Source: CAD feature listing. Evaluate the final solid. Frame: model axes, mm. Round coordinates to 2 decimals unless told otherwise and drop trailing zeros. Write each loop counter-clockwise with the first axis right and the second up, starting at its lowest first coordinate (ties: lowest second). Pieces come first, ordered by that corner, then holes. Notation, with made-up numbers: M -6.75,71.25 L 32.25,71.25 A8 ccw 32.25,78.25 Z; hole C 55,15.25 d11. An arc over 180 degrees is marked long. Answer in a Markdown table with one row per item.
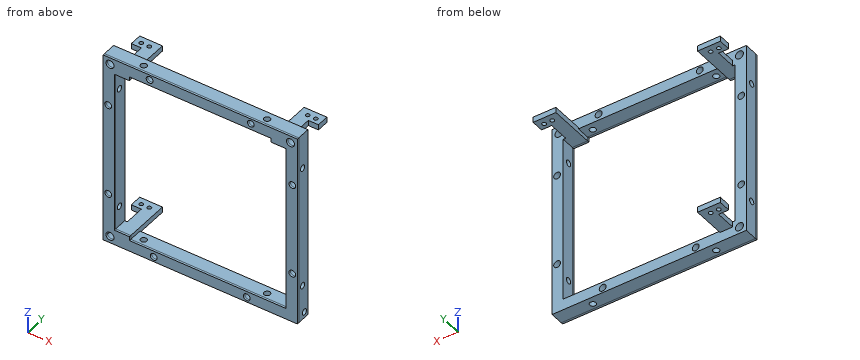
from build123d import *
from build123d.topology import SkipClean

# Parameters (mm, degrees)
SKETCH1_W                       = 96
SKETCH1_H                       = 96
SKETCH1_W_2                     = 80
SKETCH1_H_2                     = 80
BOSS_EXTRUDE1_DEPTH             = 8
SKETCH27_W                      = 82
SKETCH27_H                      = 82
CUT_EXTRUDE2_DEPTH              = 10
F_3_0_3_DIAMETER_HOLE1_D        = 3
F_3_4_3_4_DIAMETER_HOLE1_D      = 3.4
SKETCH38_W                      = 85
SKETCH38_H                      = 85
CUT_EXTRUDE4_DEPTH              = 10
F_3_0_3_DIAMETER_HOLE7_D        = 3
SKETCH44_W                      = 4
SKETCH44_H                      = 4
BOSS_EXTRUDE2_DEPTH             = 8
SKETCH45_W                      = 4
SKETCH45_H                      = 3.5
BOSS_EXTRUDE3_DEPTH             = 8
SKETCH49_W                      = 96
SKETCH49_H                      = 1.5
CUT_EXTRUDE5_DEPTH              = 146
TAP_DRILL_FOR_M4_TAP1_D         = 4
SKETCH53_W                      = 4
SKETCH53_H                      = 6.5
BOSS_EXTRUDE5_DEPTH             = 78
SKETCH57_W                      = 4
SKETCH57_H                      = 6.5
CUT_EXTRUDE6_DEPTH              = 7.5
SKETCH58_W                      = 4
SKETCH58_H                      = 6.5
BOSS_EXTRUDE7_DEPTH             = 81
SKETCH61_W                      = 32
SKETCH61_H                      = 85
CUT_EXTRUDE7_DEPTH              = 81
SKETCH66_W                      = 85
SKETCH66_H                      = 80.198
CUT_EXTRUDE8_DEPTH              = 10
SKETCH67_W                      = 85
SKETCH67_H                      = 85
CUT_EXTRUDE9_DEPTH              = 3.5
SKETCH68_W                      = 52
SKETCH68_H                      = 85
CUT_EXTRUDE10_DEPTH             = 56
SKETCH54_W                      = 6.25
SKETCH54_H                      = 2.7
BOSS_EXTRUDE8_DEPTH             = 16
CUT_EXTRUDE12_START             = -10.22
SKETCH75_W                      = 2.401
SKETCH75_H                      = 3
CUT_EXTRUDE12_DEPTH             = 72.44
SKETCH77_W                      = 2.401
SKETCH77_H                      = 3
CUT_EXTRUDE13_DEPTH             = 6.28
SKETCH78_W                      = 85
SKETCH78_H                      = 85
CUT_EXTRUDE14_DEPTH             = 6.5
SKETCH79_W                      = 85
SKETCH79_H                      = 85
SKETCH79_W_2                    = 81
SKETCH79_H_2                    = 81
BOSS_EXTRUDE12_DEPTH            = 6.5
SKETCH81_W                      = 2.7
SKETCH81_H                      = 6
BOSS_EXTRUDE13_DEPTH            = 5
TAP_DRILL_FOR_M2_TAP1_D         = 2
TAP_DRILL_FOR_M2_TAP1_DEPTH     = 5.5
TAP_DRILL_FOR_M2_TAP2_D         = 2
TAP_DRILL_FOR_M2_TAP2_DEPTH     = 5.5
TAP_DRILL_FOR_M3X0_5_TAP1_D     = 3
TAP_DRILL_FOR_M3X0_5_TAP1_DEPTH = 7.5
SKETCH88_W                      = 2
SKETCH88_H                      = 70
SKETCH88_W_2                    = 70
SKETCH88_H_2                    = 2
CUT_EXTRUDE15_DEPTH             = 10
SKETCH89_W                      = 85
SKETCH89_H                      = 81
CUT_EXTRUDE16_DEPTH             = 10
SKETCH90_W                      = 2
SKETCH90_H                      = 6.5
CUT_EXTRUDE17_DEPTH             = 7.5
SKETCH91_W                      = 96
SKETCH91_H                      = 96
SKETCH91_R                      = 1.7
SKETCH91_R_2                    = 1.64536441
SKETCH91_R_3                    = 2
BOSS_EXTRUDE14_DEPTH            = 1


with BuildPart() as part:
    # Sketch1 → Boss-Extrude1 (new body)
    with BuildSketch(Plane(origin=(0, 0, 0), x_dir=(1, 0, 0), z_dir=(0, 1, 0))):
        Rectangle(SKETCH1_W, SKETCH1_H)
        Rectangle(SKETCH1_W_2, SKETCH1_H_2, mode=Mode.SUBTRACT)
    extrude(amount=BOSS_EXTRUDE1_DEPTH)

    # Sketch27 → Cut-Extrude2 (cut)
    with BuildSketch(Plane(origin=(0, 8, 0), x_dir=(1, 0, 0), z_dir=(0, 1, 0))):
        Rectangle(SKETCH27_W, SKETCH27_H)
    extrude(amount=-CUT_EXTRUDE2_DEPTH, mode=Mode.SUBTRACT)

    # Ø3.0 (3) Diameter Hole1 (through all)
    with Locations(Plane.XY.offset(48)):
        with Locations((-30.5, 2.7), (30.5, 2.7)):
            Hole(F_3_0_3_DIAMETER_HOLE1_D / 2)

    # Ø3.4 (3.4) Diameter Hole1 (through all)
    with Locations(Plane(origin=(0, 0, 0), x_dir=(-1, 0, 0), z_dir=(0, -1, 0))):
        with Locations((-23, 45.5), (23, 45.5), (45.5, 23), (45.5, -23), (25, -45.5), (-25, -45.5), (-45.5, -23), (-45.5, 23)):
            Hole(F_3_4_3_4_DIAMETER_HOLE1_D / 2)

    # Sketch38 → Cut-Extrude4 (cut)
    with BuildSketch(Plane(origin=(0, 8, 0), x_dir=(1, 0, 0), z_dir=(0, 1, 0))):
        Rectangle(SKETCH38_W, SKETCH38_H)
    extrude(amount=-CUT_EXTRUDE4_DEPTH, mode=Mode.SUBTRACT)

    # Ø3.0 (3) Diameter Hole7 (through all)
    with Locations(Plane.ZY.offset(48)):
        with Locations((-30.5, 2.7), (30.5, 2.7)):
            Hole(F_3_0_3_DIAMETER_HOLE7_D / 2)

    # Sketch44 → Boss-Extrude2 (add)
    with BuildSketch(Plane.XZ):
        with Locations((40.5, -40.5)):
            Rectangle(SKETCH44_W, SKETCH44_H)
        with Locations((-40.5, -40.5)):
            Rectangle(SKETCH44_W, SKETCH44_H)
        with Locations((-40.5, 40.5)):
            Rectangle(SKETCH44_W, SKETCH44_H)
        with Locations((40.5, 40.5)):
            Rectangle(SKETCH44_W, SKETCH44_H)
    extrude(amount=-BOSS_EXTRUDE2_DEPTH)

    # Sketch45 → Boss-Extrude3 (add)
    with BuildSketch(Plane(origin=(0, 8, 0), x_dir=(1, 0, 0), z_dir=(0, 1, 0))):
        with Locations((-40.5, 36.75)):
            Rectangle(SKETCH45_W, SKETCH45_H)
    extrude(amount=-BOSS_EXTRUDE3_DEPTH)

    # Sketch49 → Cut-Extrude5 (cut)
    with BuildSketch(Plane(origin=(48, 0, 0), x_dir=(0, 0, -1), z_dir=(1, 0, 0))):
        with Locations((0, 7.25)):
            Rectangle(SKETCH49_W, SKETCH49_H)
    extrude(amount=-CUT_EXTRUDE5_DEPTH, mode=Mode.SUBTRACT)

    # Tap Drill for M4 Tap1 (through all)
    with Locations(Plane(origin=(0, 6.5, 0), x_dir=(1, 0, 0), z_dir=(0, 1, 0))):
        with Locations((44.6, -44.6), (-44.6, -44.6), (-44.6, 44.6)):
            Hole(TAP_DRILL_FOR_M4_TAP1_D / 2)

    # Sketch53 → Boss-Extrude5 (add)
    with BuildSketch(Plane(origin=(-38.5, 0, 0), x_dir=(0, 0, -1), z_dir=(1, 0, 0))):
        with Locations((-40.5, 3.25)):
            Rectangle(SKETCH53_W, SKETCH53_H)
    extrude(amount=BOSS_EXTRUDE5_DEPTH)

    # Sketch57 → Cut-Extrude6 (cut)
    with BuildSketch(Plane.XY.offset(-35)):
        with Locations((-40.5, 3.25)):
            Rectangle(SKETCH57_W, SKETCH57_H)
    extrude(amount=-CUT_EXTRUDE6_DEPTH, mode=Mode.SUBTRACT)

    # Sketch58 → Boss-Extrude7 (add)
    with BuildSketch(Plane.ZY.offset(-38.5)):
        with Locations((-40.5, 3.25)):
            Rectangle(SKETCH58_W, SKETCH58_H)
    extrude(amount=BOSS_EXTRUDE7_DEPTH)

    # Sketch61 → Cut-Extrude7 (cut)
    with BuildSketch(Plane(origin=(0, 6.5, 0), x_dir=(1, 0, 0), z_dir=(0, 1, 0))):
        Rectangle(SKETCH61_W, SKETCH61_H)
    extrude(amount=-CUT_EXTRUDE7_DEPTH, mode=Mode.SUBTRACT)

    # Sketch66 → Cut-Extrude8 (cut)
    with BuildSketch(Plane(origin=(0, 6.5, 0), x_dir=(1, 0, 0), z_dir=(0, 1, 0))):
        Rectangle(SKETCH66_W, SKETCH66_H)
    extrude(amount=-CUT_EXTRUDE8_DEPTH, mode=Mode.SUBTRACT)

    # Sketch67 → Cut-Extrude9 (cut)
    with BuildSketch(Plane.XZ):
        Rectangle(SKETCH67_W, SKETCH67_H)
    extrude(amount=-CUT_EXTRUDE9_DEPTH, mode=Mode.SUBTRACT)

    # Sketch68 → Cut-Extrude10 (cut)
    with BuildSketch(Plane(origin=(0, 6.5, 0), x_dir=(1, 0, 0), z_dir=(0, 1, 0))):
        Rectangle(SKETCH68_W, SKETCH68_H)
    extrude(amount=-CUT_EXTRUDE10_DEPTH, mode=Mode.SUBTRACT)

    # Sketch54 → Boss-Extrude8 (add)
    with BuildSketch(Plane(origin=(0, 6.5, 0), x_dir=(1, 0, 0), z_dir=(0, 1, 0))):
        with Locations((-38.125, -41.85)):
            Rectangle(SKETCH54_W, SKETCH54_H)
    boss_extrude8 = extrude(amount=BOSS_EXTRUDE8_DEPTH)

    # Mirror1: Boss-Extrude8 across plane
    add(boss_extrude8.mirror(Plane(origin=(0, 0, 0), x_dir=(0, 0, 1), z_dir=(1, 0, 0))))

    # Sketch75 → Cut-Extrude12 (cut)
    with BuildSketch(Plane.ZY.offset(-26).offset(CUT_EXTRUDE12_START)):
        with Locations((41.2995, 5)):
            Rectangle(SKETCH75_W, SKETCH75_H)
    cut_extrude12 = extrude(amount=CUT_EXTRUDE12_DEPTH, mode=Mode.SUBTRACT)

    # Mirror2: Boss-Extrude8 across plane
    add(boss_extrude8.mirror(Plane.XY))

    # Mirror3: Cut-Extrude12 across plane
    add(cut_extrude12.mirror(Plane.XY), mode=Mode.SUBTRACT)

    # Sketch77 → Cut-Extrude13 (cut)
    with BuildSketch(Plane.ZY.offset(-36.22)):
        with Locations((-41.2995, 5)):
            Rectangle(SKETCH77_W, SKETCH77_H)
    extrude(amount=-CUT_EXTRUDE13_DEPTH, mode=Mode.SUBTRACT)

    # Sketch78 → Cut-Extrude14 (cut)
    with BuildSketch(Plane.XZ):
        Rectangle(SKETCH78_W, SKETCH78_H)
    extrude(amount=-CUT_EXTRUDE14_DEPTH, mode=Mode.SUBTRACT)

    # Sketch79 → Boss-Extrude12 (add)
    with BuildSketch(Plane.XZ):
        Rectangle(SKETCH79_W, SKETCH79_H)
        Rectangle(SKETCH79_W_2, SKETCH79_H_2, mode=Mode.SUBTRACT)
    extrude(amount=-BOSS_EXTRUDE12_DEPTH)

    # Sketch81 → Boss-Extrude13 (add)
    with BuildSketch(Plane.ZY.offset(41.25)):
        with Locations((41.85, 19.5)):
            Rectangle(SKETCH81_W, SKETCH81_H)
    boss_extrude13 = extrude(amount=BOSS_EXTRUDE13_DEPTH)

    # Mirror4: Boss-Extrude13 across plane
    add(boss_extrude13.mirror(Plane.XY))

    # Mirror5: Boss-Extrude13 across plane
    add(boss_extrude13.mirror(Plane(origin=(0, 0, 0), x_dir=(0, 0, 1), z_dir=(1, 0, 0))))

    # Tap Drill for M2 Tap1
    with Locations(Plane(origin=(0, 0, 40.5), x_dir=(-1, 0, 0), z_dir=(0, 0, -1))):
        with Locations((39.147345831, 19.1), (43.147345831, 19.1), (-39.15, 19.1), (-43.15, 19.1)):
            Hole(TAP_DRILL_FOR_M2_TAP1_D / 2, depth=TAP_DRILL_FOR_M2_TAP1_DEPTH)

    # Tap Drill for M2 Tap2
    with Locations(Plane.XY.offset(-40.5)):
        with Locations((-39.147345831, 19.1), (-43.147345831, 19.1)):
            Hole(TAP_DRILL_FOR_M2_TAP2_D / 2, depth=TAP_DRILL_FOR_M2_TAP2_DEPTH)

    # Tap Drill for M3x0.5 Tap1
    with Locations(Plane(origin=(48, 0, 0), x_dir=(0, 0, -1), z_dir=(1, 0, 0))):
        with Locations((45, 4)):
            Hole(TAP_DRILL_FOR_M3X0_5_TAP1_D / 2, depth=TAP_DRILL_FOR_M3X0_5_TAP1_DEPTH)

    # Sketch88 → Cut-Extrude15 (cut)
    with BuildSketch(Plane(origin=(0, 6.5, 0), x_dir=(1, 0, 0), z_dir=(0, 1, 0))):
        with Locations((41.5, 0)):
            Rectangle(SKETCH88_W, SKETCH88_H)
        with Locations((0, -41.5)):
            Rectangle(SKETCH88_W_2, SKETCH88_H_2)
        with Locations((-41.5, 0)):
            Rectangle(SKETCH88_W, SKETCH88_H)
        with Locations((0, 41.5)):
            Rectangle(SKETCH88_W_2, SKETCH88_H_2)
    extrude(amount=-CUT_EXTRUDE15_DEPTH, mode=Mode.SUBTRACT)

    # Sketch89 → Cut-Extrude16 (cut)
    with BuildSketch(Plane(origin=(0, 6.5, 0), x_dir=(1, 0, 0), z_dir=(0, 1, 0))):
        Rectangle(SKETCH89_W, SKETCH89_H)
    extrude(amount=-CUT_EXTRUDE16_DEPTH, mode=Mode.SUBTRACT)

    # Sketch90 → Cut-Extrude17 (cut)
    with BuildSketch(Plane.ZY.offset(-35)):
        with Locations((-41.5, 3.25)):
            Rectangle(SKETCH90_W, SKETCH90_H)
    extrude(amount=-CUT_EXTRUDE17_DEPTH, mode=Mode.SUBTRACT)

    # Sketch91 → Boss-Extrude14 (add)
    with SkipClean():  # the faces are left unmerged after this step: merging them gives an invalid solid
        with BuildSketch(Plane.XZ):
            Rectangle(SKETCH91_W, SKETCH91_H)
            with Locations(Location((-25, 45.5, 0), (0, 0, 270))):
                Circle(SKETCH91_R, mode=Mode.SUBTRACT)
            with Locations(Location((25, 45.5, 0), (0, 0, 270))):
                Circle(SKETCH91_R_2, mode=Mode.SUBTRACT)
            with Locations(Location((44.6, 44.6, 0), (0, 0, 90))):
                Circle(SKETCH91_R_3, mode=Mode.SUBTRACT)
            with Locations(Location((45.5, 23, 0), (0, 0, 270))):
                Circle(SKETCH91_R, mode=Mode.SUBTRACT)
            with Locations(Location((45.5, -23, 0), (0, 0, 270))):
                Circle(SKETCH91_R, mode=Mode.SUBTRACT)
            with Locations(Location((23, -45.5, 0), (0, 0, 270))):
                Circle(SKETCH91_R, mode=Mode.SUBTRACT)
            with Locations(Location((-23, -45.5, 0), (0, 0, 270))):
                Circle(SKETCH91_R, mode=Mode.SUBTRACT)
            with Locations(Location((-45.5, -23, 0), (0, 0, 270))):
                Circle(SKETCH91_R, mode=Mode.SUBTRACT)
            with Locations(Location((-44.6, -44.6, 0), (0, 0, 90))):
                Circle(SKETCH91_R_3, mode=Mode.SUBTRACT)
            with Locations(Location((-45.5, 23, 0), (0, 0, 270))):
                Circle(SKETCH91_R, mode=Mode.SUBTRACT)
            with Locations(Location((-44.6, 44.6, 0), (0, 0, 90))):
                Circle(SKETCH91_R_3, mode=Mode.SUBTRACT)
            Polygon((42.5, -42.5), (-35, -42.5), (-35, -40.5), (-42.5, -40.5), (-42.5, 40.5), (-35, 40.5), (-35, 42.5), (35, 42.5), (35, 40.5), (42.5, 40.5), align=None, mode=Mode.SUBTRACT)
        extrude(amount=BOSS_EXTRUDE14_DEPTH)


solid = part.part
Q1. Material intervals for probe 1 along Z at (x, y) = (25, 3.5); probe 2 along Z at (x, y) = (-17.5, 5.75); probe 3 along X at (y, z) = (4, -45.5), sorted ascending.
Solutions:
| item | result |
|---|---|
| probe 1 | z = -48 to -42.5, 42.5 to 43.8, 47.2 to 48 |
| probe 2 | z = -48 to -42.5, 42.5 to 48 |
| probe 3 | x = -48 to -46.39, -42.81 to -31.25, -29.75 to -24.7, -21.3 to 21.3, 24.7 to 29.75, 31.25 to 40.5 |
Q2. Section D-D (z = -23). Return loops of the section in (x, y).
Solutions:
| item | result |
|---|---|
| outline | M -48,-1 L -47.2,-1 L -47.2,6.5 L -48,6.5 Z; M -43.8,-1 L -42.5,-1 L -42.5,6.5 L -43.8,6.5 Z; M 42.5,-1 L 43.8,-1 L 43.8,6.5 L 42.5,6.5 Z; M 47.2,-1 L 48,-1 L 48,6.5 L 47.2,6.5 Z |
Q3. Section A-A (y = 9). Return loops of the section in (x, z), and give its area (3 significant figures).
Solutions:
| item | result |
|---|---|
| outline | M -41.25,-43.2 L -35,-43.2 L -35,-40.5 L -41.25,-40.5 Z; M -41.25,40.5 L -35,40.5 L -35,43.2 L -41.25,43.2 Z; M 35,40.5 L 41.25,40.5 L 41.25,43.2 L 35,43.2 Z |
| area | 50.6 mm2 |
Q4. Contact query for flat-ended pins moving along their axis: pin 1 Ø5 at (y, z) = (2.7, -30.5) entering from +X; pin 2 Ø5.5 at (x, z) = (-45.5, -23) entering from +Y; pin 3 Ø2 at (y, z) = (12, 42) entering from -X. Output: stop coordinate, or through.
Solutions:
| item | result |
|---|---|
| pin 1 | stops at x = 48 |
| pin 2 | stops at y = 6.5 |
| pin 3 | stops at x = -41.25 |
Q5. Section C-C (x = 5.5). Return loops of the section in (y, z).
Solutions:
| item | result |
|---|---|
| outline | M -1,-48 L 6.5,-48 L 6.5,-42.5 L -1,-42.5 Z; M -1,42.5 L 6.5,42.5 L 6.5,48 L -1,48 Z |
Q6. Section B-B (z = -1). Return loops of the section in (x, y), and give its area (3 significant figures).
Solutions:
| item | result |
|---|---|
| outline | M -48,-1 L -42.5,-1 L -42.5,6.5 L -48,6.5 Z; M 42.5,-1 L 48,-1 L 48,6.5 L 42.5,6.5 Z |
| area | 82.5 mm2 |
